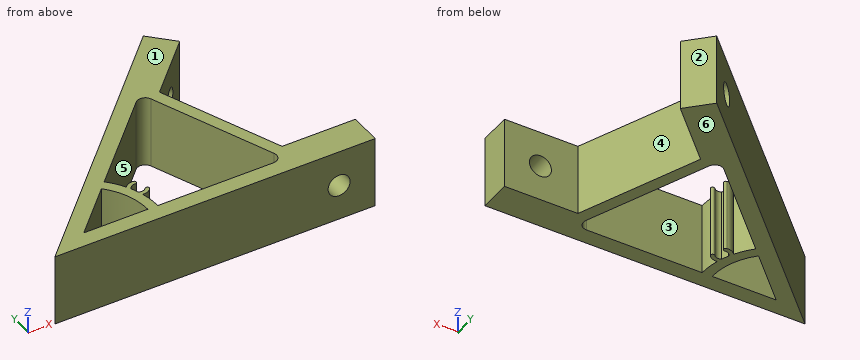
from build123d import *

# Parameters (mm, degrees)
EXTRUDE_1_DEPTH     = 18
SKETCH_2_R          = 2.75
CUT_EXTRUDE_1_DEPTH = 28
SKETCH_3_R          = 2.75
CUT_EXTRUDE_2_DEPTH = 28


with BuildPart() as part:
    # 草图1 → 凸台-拉伸1 (new body)
    # profile 1 of 2: a face of its own
    with BuildSketch(Plane.XY):
        Polygon((80, 0), (80, 8), (61.629823519, 8), (49.235720383, 37.922011884), (62.225396744, 50.911688245), (56.568542495, 56.568542495), (0, 0), align=None)
        with BuildLine():
            ThreePointArc((46.428217999, 36.860544425), (44.970639578, 38.056748121), (43.166245372, 37.509391123))
            Line((43.166245372, 37.509391123), (9.656854249, 4))
            Line((9.656854249, 4), (57.046289642, 4))
            ThreePointArc((57.046289642, 4), (58.709228866, 4.888859534), (58.894048707, 6.765366865))
            Line((58.894048707, 6.765366865), (46.428217999, 36.860544425))
        make_face(mode=Mode.SUBTRACT)
    # profile 2 of 2: a face of its own
    with BuildSketch(Plane.XY):
        with BuildLine():
            Line((25.656854249, 4), (28.156854249, 4))
            ThreePointArc((28.156854249, 4), (27.980871323, 6.54566264), (27.456270652, 9.042893586))
            ThreePointArc((27.456270652, 9.042893586), (28.736340858, 9.197193956), (29.769286429, 9.968823258))
            ThreePointArc((29.769286429, 9.968823258), (29.686739249, 10.671095259), (28.984467248, 10.588548079))
            ThreePointArc((28.984467248, 10.588548079), (28.105812081, 10.048151022), (27.085956296, 10.202934937))
            ThreePointArc((27.085956296, 10.202934937), (26.748625601, 11.079643499), (26.367227854, 11.93809889))
            ThreePointArc((26.367227854, 11.93809889), (26.978926039, 12.768694587), (27.982347489, 13.007879191))
            ThreePointArc((27.982347489, 13.007879191), (28.537298455, 13.446090814), (28.099086832, 14.001041779))
            ThreePointArc((28.099086832, 14.001041779), (26.823059701, 13.816263273), (25.808806541, 13.020223788))
            ThreePointArc((25.808806541, 13.020223788), (24.413946296, 15.156981417), (22.738329701, 17.081475452))
            Line((22.738329701, 17.081475452), (20.970562748, 15.313708499))
            ThreePointArc((20.970562748, 15.313708499), (24.43892677, 10.122934918), (25.656854249, 4))
        make_face()
    extrude(amount=EXTRUDE_1_DEPTH)

    # 草图2 → 切除-拉伸1 (cut)
    with BuildSketch(Plane(origin=(0, 8, 0), x_dir=(1, 0, 0), z_dir=(0, 1, 0))):
        with Locations(Location((71, -9, 0), (0, 0, 180))):
            Circle(SKETCH_2_R)
    extrude(amount=-CUT_EXTRUDE_1_DEPTH, mode=Mode.SUBTRACT)

    # 草图3 → 切除-拉伸2 (cut)
    with BuildSketch(Plane(origin=(5.656854249, -5.656854249, 0), x_dir=(0, 0, -1), z_dir=(0.7071067811865488, -0.7071067811865464, 0))):
        with Locations(Location((-9, 71, 0), (0, 0, 90))):
            Circle(SKETCH_3_R)
    extrude(amount=-CUT_EXTRUDE_2_DEPTH, mode=Mode.SUBTRACT)


solid = part.part
Geometry: final body of the model. Coordinates: model frame, mm. Face numbers are marked on the shaded views. A direction names the side the tool comes from. Give positions to 0.01 mm unless a question says otherwise; leave off trailing zeros. Loops run counter-clockwise (first coordinate to the right, second up) from the corner with the lowest first, then second, coordinate; pieces in that order, holes last. Notation, with made-up numbers: (-31, 17.25) - (-11, 17.25) arc R29 ccw to (-11, 50.25) - close; hole circle Ø5 at (20.25, 23.25). An arc over 180 degrees is marked (long way). Answer as CSV lines item,"result". Start each with the question number.
1. Section A-A, the plane x = 71. Return loops of the section in (y, z), plus the area to 3 significant figures.
2. Section C-C, the plane y = 28. Return loops of the section in (x, z), plus the area to 3 significant figures.
3. Draft query along Y for the marked faces 1, 2 and 3. Return one class per face: released by +Y, released by -Y, zero draft, split by the parting line, or undercut.
4. Section D-D, the plane z = 2.5. Return loops of the section in (x, y).
5. Reachability of the marked faces 4, 5 and 6 from +Z, -Z, +X, -X, +Y, -Y: full face, straight path, thin tool, end or side. Return the list, or none.
6. Ray query, L1, parallel to Z at x = 71, y = 4.25; L2, parallel to Y at x = 29, z = 11.75; L3, parallel to Y at x = 56, z = 6. Return the intervals inside material, ascending.
7. Pin query (flat end, axial travel): P1, Ø6, axis at x = 16, z = 9, coming from the +Y side; P2, Ø5, axis at x = 49, z = 5, coming from the +Y side; P3, Ø5, axis at y = 22.5, z = 13, coming from the +X side. Return the tip coordinate at first contact, or that it passes through.
8. Section B-B, the plane z = 9. Give the number of separate pieces and of enclosed holes in the cut face, plus the area to 3 significant figures.
Answers:
1,outline,"(0, 0) - (8, 0) - (8, 6.25) - (0, 6.25) - close; (0, 11.75) - (8, 11.75) - (8, 18) - (0, 18) - close"
1,area,"100 mm2"
2,outline,"(28, 0) - (33.66, 0) - (33.66, 18) - (28, 18) - close; (50.1, 0) - (53.35, 0) - (53.35, 18) - (50.1, 18) - close"
2,area,"160 mm2"
3,face 1,"zero draft"
3,face 2,"released by +Y"
3,face 3,"undercut"
4,outline,"(0, 0) - (80, 0) - (80, 8) - (61.63, 8) - (49.24, 37.92) - (62.23, 50.91) - (56.57, 56.57) - close; hole (9.66, 4) - (25.66, 4) arc R16 ccw to (20.97, 15.31) - close; hole (22.74, 17.08) arc R18.5 cw to (25.81, 13.02) arc R2.5 cw to (28.1, 14) arc R0.5 cw to (27.98, 13.01) arc R1.5 ccw to (26.37, 11.94) arc R18.5 cw to (27.09, 10.2) arc R1.5 ccw to (28.98, 10.59) arc R0.5 cw to (29.77, 9.97) arc R2.5 cw to (27.46, 9.04) arc R18.5 cw to (28.16, 4) - (57.05, 4) arc R2 ccw to (58.89, 6.77) - (46.43, 36.86) arc R2 ccw to (43.17, 37.51) - close"
5,face 4,"+Z, -Z, +X"
5,face 5,"+Z, -Z"
5,face 6,"-Z, +X, -X, +Y, -Y"
6,L1,"z = 0 to 6.25, 11.75 to 18"
6,L2,"y = 0 to 4, 9.32 to 10.61, 23.34 to 29"
6,L3,"y = 0 to 4, 13.75 to 21.59, 44.69 to 56"
7,P1,"stops at y = 19"
7,P2,"stops at y = 51.5"
7,P3,"stops at x = 56.66"
8,separate pieces,"3"
8,enclosed holes,"2"
8,area,"817 mm2"
